Print and shaded views of the part. All mm, measured from the part's lowest x, y and z. Coordinates: 2 decimals unless noted, no trailing zeros. Order: outer loops, then holes, each group sorted by start corner. A loop starts at its lowest first (then second) coordinate and runs counter-clockwise, first axis right, second up. Notation, with made-up numbers: M 51,15.5 L 105,15.5 A22 ccw 105,42.5 Z; hole C 15,-0.5 d8. An arc over 180 degrees is marked long. One line per item, written item: value.
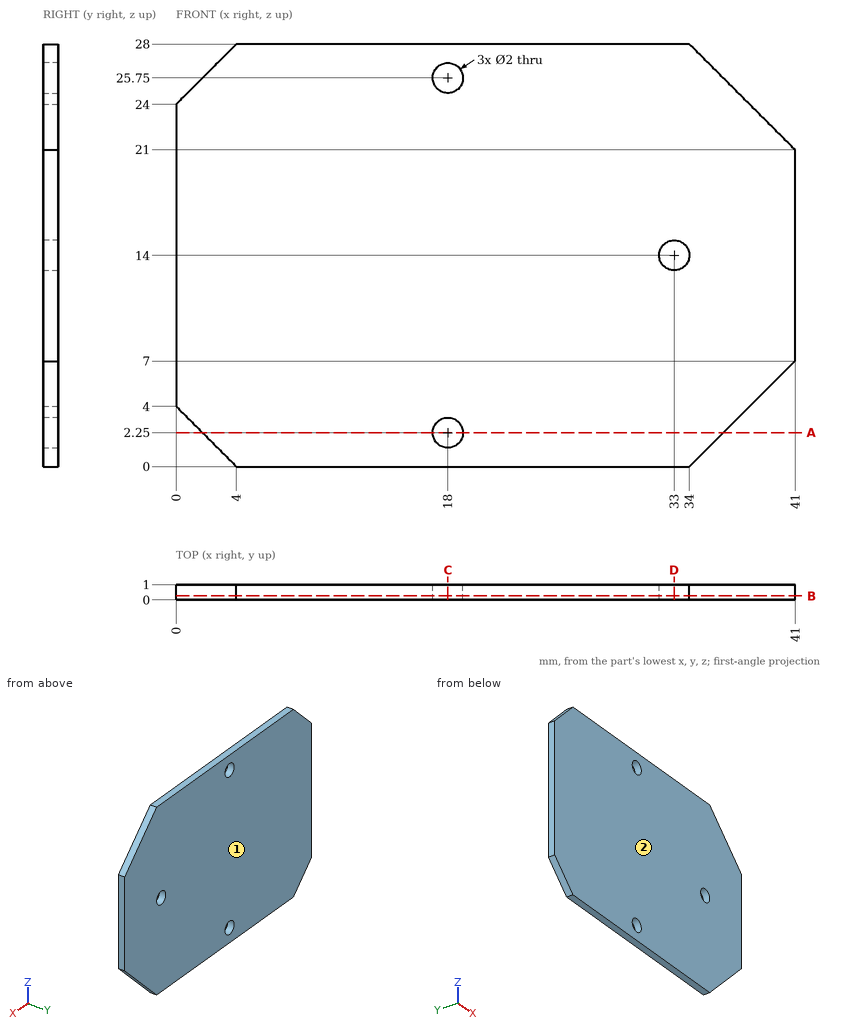
Q1. Mould opens along Y. For the marked faces 1 and 2 say: released by +Y, released by -Y, zero draft, split by the parting line, or undercut.
Recorded:
face 1: released by +Y
face 2: released by -Y
Q2. Slice it at A-A (z = 2.25). List the corners of the cut face in (x, y).
Recorded:
outline: M 1.75,0 L 17,0 L 17,1 L 1.75,1 Z; M 19,0 L 36.25,0 L 36.25,1 L 19,1 Z
Q3. Slice it at D-D (x = 33). List the corners of the cut face in (y, z).
Recorded:
outline: M 0,0 L 1,0 L 1,13 L 0,13 Z; M 0,15 L 1,15 L 1,28 L 0,28 Z
Q4. Slice it at B-B (y = 0.25). List the corners of the cut face in (x, z).
Recorded:
outline: M 0,4 L 4,0 L 34,0 L 41,7 L 41,21 L 34,28 L 4,28 L 0,24 Z; hole C 18,2.25 d2; hole C 18,25.75 d2; hole C 33,14 d2
Q5. Drill centre lines: line 1 along Z through (x, y) = (33, 0.15); line 2 along X through (y, z) = (0.75, 14); line 3 along X through (y, z) = (0.6, 25.75). Where is each one in solid material? Low to high.
Recorded:
line 1: z = 0 to 13, 15 to 28
line 2: x = 0 to 32, 34 to 41
line 3: x = 1.75 to 17, 19 to 36.25
Q6. Slice it at C-C (x = 18). List the corners of the cut face in (y, z).
Recorded:
outline: M 0,0 L 1,0 L 1,1.25 L 0,1.25 Z; M 0,3.25 L 1,3.25 L 1,24.75 L 0,24.75 Z; M 0,26.75 L 1,26.75 L 1,28 L 0,28 Z
